CAD build for the part. Positions are in the model's coordinates, mm. A direction names the side the tool comes from. Coordinates: 2 decimals unless noted, no trailing zeros. Order: outer loops, then holes, each group sorted by start corner. A loop starts at its lowest first (then second) coordinate and runs counter-clockwise, first axis right, second up. Notation, with made-up numbers: (-37, 46) - (-19, 46) arc R5 ccw to (-19, 55) - close; hole circle Ø7 at (-12.5, -35.75). An arc over 180 degrees is marked (long way). Use one line per item in the form item = value.
```python
from build123d import *

# Parameters (mm, degrees)
SKETCH_W        = 143
SKETCH_H        = 96
PAD_DEPTH       = 15.6
SKETCH001_W     = 133
SKETCH001_H     = 86
POCKET_DEPTH    = 13.6
SKETCH002_W     = 6
SKETCH002_H     = 6
PAD001_DEPTH    = 12
SKETCH003_R     = 1
POCKET001_DEPTH = 11.6
SKETCH004_W     = 12
SKETCH004_H     = 6
POCKET002_DEPTH = 5.001
SKETCH005_W     = 133
SKETCH005_H     = 2
PAD002_DEPTH    = 12


with BuildPart() as part:
    # Sketch → Pad (new body)
    with BuildSketch(Plane.XY):
        with Locations((71.5, 48)):
            Rectangle(SKETCH_W, SKETCH_H)
    extrude(amount=-PAD_DEPTH)

    # Sketch001 (on Face5 of Pad) → Pocket (cut)
    with BuildSketch(Plane.XY):
        with Locations((71.5, 48)):
            Rectangle(SKETCH001_W, SKETCH001_H)
    extrude(amount=-POCKET_DEPTH, mode=Mode.SUBTRACT)

    # Sketch002 (on Face11 of Pocket) → Pad001 (join)
    with BuildSketch(Plane.XY.offset(-13.6)):
        with Locations((8, 8)):
            Rectangle(SKETCH002_W, SKETCH002_H)
        with Locations((135, 8)):
            Rectangle(SKETCH002_W, SKETCH002_H)
        with Locations((8, 52)):
            Rectangle(SKETCH002_W, SKETCH002_H)
        with Locations((135, 52)):
            Rectangle(SKETCH002_W, SKETCH002_H)
        with Locations((8, 88)):
            Rectangle(SKETCH002_W, SKETCH002_H)
        with Locations((135, 88)):
            Rectangle(SKETCH002_W, SKETCH002_H)
    extrude(amount=PAD001_DEPTH)

    # Sketch003 (on Face18 of Pad001) → Pocket001 (cut)
    with BuildSketch(Plane.XY.offset(-1.6)):
        with Locations((8.5, 87.5)):
            Circle(SKETCH003_R)
        with Locations((8.5, 52)):
            Circle(SKETCH003_R)
        with Locations((8.5, 8.5)):
            Circle(SKETCH003_R)
        with Locations((134.5, 87.5)):
            Circle(SKETCH003_R)
        with Locations((134.5, 52)):
            Circle(SKETCH003_R)
        with Locations((134.5, 8.5)):
            Circle(SKETCH003_R)
    extrude(amount=-POCKET001_DEPTH, mode=Mode.SUBTRACT)

    # Sketch004 (on Face9 of Pocket001) → Pocket002 (cut, through all)
    with BuildSketch(Plane(origin=(138, 0, 0), x_dir=(0, -1, 0), z_dir=(-1, 0, 0))):
        with Locations((-70.39, -10.6)):
            Rectangle(SKETCH004_W, SKETCH004_H)
    extrude(amount=-POCKET002_DEPTH, mode=Mode.SUBTRACT)

    # Sketch005 (on Face17 of Pocket002) → Pad002 (join)
    with BuildSketch(Plane.XY.offset(-13.6)):
        with Locations((71.5, 12.5)):
            Rectangle(SKETCH005_W, SKETCH005_H)
        with Locations((71.5, 22.5)):
            Rectangle(SKETCH005_W, SKETCH005_H)
        with Locations((71.5, 32.5)):
            Rectangle(SKETCH005_W, SKETCH005_H)
        with Locations((71.5, 42.5)):
            Rectangle(SKETCH005_W, SKETCH005_H)
    extrude(amount=PAD002_DEPTH)


solid = part.part
```
Item 1: 3-axis set-ups, long thin cutter, end or side, ignore diameter. For faces 1 (the face through (66, 2, 0)), 2 (the face through (11, 8, -8)), 3 (the face through (140, 76.39, -11)): which of +Z, -Z, +X, -X, +Y, -Y reach the whole face in a straight line?
Derived:
face_1 = +Z, +X, -X, +Y, -Y
face_2 = +Z
face_3 = +X
Item 2: Cut at A-A, the plane x = 26.5. Write the cut outline in (y, z).
Derived:
outline = (0, -15.6) - (96, -15.6) - (96, 0) - (91, 0) - (91, -13.6) - (43.5, -13.6) - (43.5, -1.6) - (41.5, -1.6) - (41.5, -13.6) - (33.5, -13.6) - (33.5, -1.6) - (31.5, -1.6) - (31.5, -13.6) - (23.5, -13.6) - (23.5, -1.6) - (21.5, -1.6) - (21.5, -13.6) - (13.5, -13.6) - (13.5, -1.6) - (11.5, -1.6) - (11.5, -13.6) - (5, -13.6) - (5, 0) - (0, 0) - close
Item 3: Drop flat-ended pins along their axis: pin 1 (5 mm diameter, centred on x = 112.5, y = 24, fed in from +Z); pin 2 (2 mm diameter, centred on x = 32, y = 38.5, fed in from +Z). Give the stop position or say it passes through.
Derived:
pin_1 = -1.6
pin_2 = -13.6
Item 4: Cut at B-B, the plane y = 83. Write the cut outline in (x, z), plus the area to 3 significant figures.
Derived:
outline = (0, -15.6) - (143, -15.6) - (143, 0) - (138, 0) - (138, -13.6) - (5, -13.6) - (5, 0) - (0, 0) - close
area = 422 mm²
Item 5: Cut at C-C, the plane z = -10. State how many separate pieces and enclosed holes the cut face has, plus the area to 3 significant figures.
Derived:
separate_pieces = 1
enclosed_holes = 10
area = 3,490 mm²
Item 6: Drill centre lines: line 1 (Y direction, x = 13, z = -1.75); line 2 (X direction, y = 61, z = -3); line 3 (X direction, y = 87.5, z = -8.5). Where is each one in solid material? Low to high. Write a range as [from, to].
Derived:
line_1 = [0, 5], [11.5, 13.5], [21.5, 23.5], [31.5, 33.5], [41.5, 43.5], [91, 96]
line_2 = [0, 5], [138, 143]
line_3 = [0, 7.5], [9.5, 11], [132, 133.5], [135.5, 143]
Item 7: Two-plate mould, pull along Y, no slides. Class faces 4 (the face through (70, 0, -8)), 5 (the face through (71, 41.5, -8)), 6 (the face through (70, 96, -8)): +Y half, -Y half, draft (parallel to the pull), parting line (faces both ways), or undercut.
Derived:
face_4 = -Y half
face_5 = undercut
face_6 = +Y half
